The listing builds one solid part. Answer for the finished solid, in the listing's coordinates (mm). Face numbers are marked on the shaded views. A direction names the side the tool comes from. Coordinates: 2 decimals unless noted, no trailing zeros. Write each loop counter-clockwise with the first axis right and the second up, starting at its lowest first coordinate (ties: lowest second). Pieces come first, ordered by that corner, then holes.
(1) Which of the six approach directions +Z, -Z, +X, -X, +Y, -Y give full straight-line access (tool end or side, diameter ignored) to the marked faces 1, 2 and 3?
(2) Straight lines are drawn through the part: line 1 (Y direction, x = 14.5, z = 1.2); line 2 (X direction, y = 11, z = 2.25); line 3 (Z direction, x = 3.5, y = 65). For each, find the intervals that lie inside material, in ascending order.
(3) The part is cut by section D-D on y = 46.5. Determine the outline of the cut face in (x, z), plus the area to 3 significant figures.
(4) The part is cut by section A-A on z = 1.7. Determine the outline of the cut face in (x, y), plus the area to 3 significant figures.
(5) Given P1, Ø0.6, axis at x = -1, z = 0.5, coming from the +Y side; P2, Ø10, axis at x = 6.5, y = 68, coming from the -Z side; P3, Ø1.5, axis at y = 42.5, z = 1.5, coming from the +X side, each flat-ended and moving along its own axis, determine where each tip first touches the part or whether it passes through.
(6) The part is cut by section C-C on x = 0. Determine the outline of the cut face in (y, z), plus the area to 3 significant figures.
(7) The part is cut by section B-B on y = 74.5. Determine the outline of the cut face in (x, z).
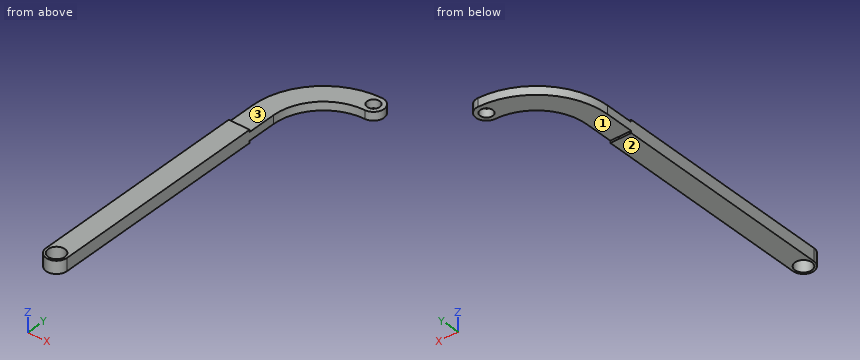
from build123d import *

# Parameters (mm, degrees)
SKETCH_1_R               = 2
SKETCH_1_R_2             = 1.5
EXTRUDE_1_DEPTH          = 3
SKETCH_2_W               = 0.5
SKETCH_2_H               = 23.89994555
SKETCH_2_W_2             = 0.589580916
CUT_EXTRUDE_1_DEPTH      = 18
CUT_EXTRUDE_1_DEPTH_BACK = 3.5


with BuildPart() as part:
    # 草图1 → 凸台-拉伸1 (new body)
    with BuildSketch(Plane.XY):
        with BuildLine():
            Line((-2.5, 0), (-2.5, 60))
            ThreePointArc((-2.5, 60), (2.47918472, 72.02081528), (14.5, 77))
            ThreePointArc((14.5, 77), (17, 74.5), (14.5, 72))
            ThreePointArc((14.5, 72), (6.014718626, 68.485281374), (2.5, 60))
            Line((2.5, 60), (2.5, 0))
            ThreePointArc((2.5, 0), (0, -2.5), (-2.5, 0))
        make_face()
        Circle(SKETCH_1_R, mode=Mode.SUBTRACT)
        with Locations((14.5, 74.5)):
            Circle(SKETCH_1_R_2, mode=Mode.SUBTRACT)
    extrude(amount=EXTRUDE_1_DEPTH)

    # 草图2 → 切除-拉伸1 (cut, two sides)
    with BuildSketch(Plane(origin=(0, 0, 0), x_dir=(0, 0, -1), z_dir=(1, 0, 0))) as cut_extrude_1_sk:
        with Locations((-0.25, 65.050027225)):
            Rectangle(SKETCH_2_W, SKETCH_2_H)
        with Locations((-2.790044711, 65.050027225)):
            Rectangle(SKETCH_2_W_2, SKETCH_2_H)
    extrude(amount=CUT_EXTRUDE_1_DEPTH, mode=Mode.SUBTRACT)
    extrude(cut_extrude_1_sk.sketch, amount=-CUT_EXTRUDE_1_DEPTH_BACK, mode=Mode.SUBTRACT)


solid = part.part
Model answer:
1. face 1: -Z, +X, -X, +Y
1. face 2: -Z, +X, -X, +Y, -Y
1. face 3: +Z, +X, -X, +Y
2. line 1: y = 72 to 73, 76 to 77
2. line 2: x = -2.5 to 2.5
2. line 3: z = 0.5 to 2.5
3. outline: (-2.5, 0) - (2.5, 0) - (2.5, 3) - (-2.5, 3) - close
3. area: 15.0 mm2
4. outline: (-2.5, 0) arc R2.5 ccw to (2.5, 0) - (2.5, 60) arc R12 cw to (14.5, 72) arc R2.5 ccw to (14.5, 77) arc R17 ccw to (-2.5, 60) - close; hole circle Ø4 at (0, 0); hole circle Ø3 at (14.5, 74.5)
4. area: 414 mm2
5. P1: stops at y = 67.61
5. P2: stops at z = 0.5
5. P3: stops at x = 2.5
6. outline: (-2.5, 0) - (-2, 0) - (-2, 3) - (-2.5, 3) - close; (2, 0) - (53.1, 0) - (53.1, 0.5) - (68.87, 0.5) - (68.87, 2.5) - (53.1, 2.5) - (53.1, 3) - (2, 3) - close
6. area: 186 mm2
7. outline: (5.63, 0.5) - (13, 0.5) - (13, 2.5) - (5.63, 2.5) - close; (16, 0.5) - (17, 0.5) - (17, 2.5) - (16, 2.5) - close
